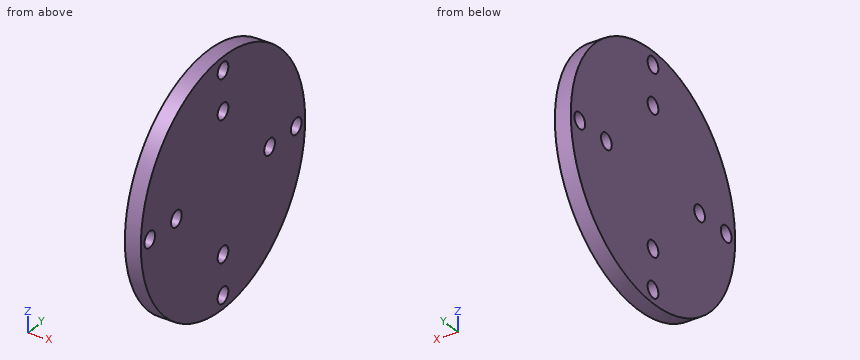
from build123d import *

# Parameters (mm, degrees)
SKETCH1_R           = 23
SKETCH1_R_2         = 1.5
BOSS_EXTRUDE1_DEPTH = 3


with BuildPart() as part:
    # Sketch1 → Boss-Extrude1 (new body)
    with BuildSketch(Plane(origin=(0, 0, 0), x_dir=(0, 0, -1), z_dir=(1, 0, 0))):
        with Locations((0, 16.5)):
            Circle(SKETCH1_R)
        with Locations((0, -4)):
            Circle(SKETCH1_R_2, mode=Mode.SUBTRACT)
        with Locations((0, 3.46)):
            Circle(SKETCH1_R_2, mode=Mode.SUBTRACT)
        with Locations((-13.04, 16.5)):
            Circle(SKETCH1_R_2, mode=Mode.SUBTRACT)
        with Locations((-20.5, 16.5)):
            Circle(SKETCH1_R_2, mode=Mode.SUBTRACT)
        with Locations((0, 29.54)):
            Circle(SKETCH1_R_2, mode=Mode.SUBTRACT)
        with Locations((0, 37)):
            Circle(SKETCH1_R_2, mode=Mode.SUBTRACT)
        with Locations((13.04, 16.5)):
            Circle(SKETCH1_R_2, mode=Mode.SUBTRACT)
        with Locations((20.5, 16.5)):
            Circle(SKETCH1_R_2, mode=Mode.SUBTRACT)
    extrude(amount=BOSS_EXTRUDE1_DEPTH)


solid = part.part
The listing builds one solid part. Answer for the finished solid, in the listing's coordinates (mm). Coordinates: 2 decimals unless noted, no trailing zeros. Order: outer loops, then holes, each group sorted by start corner. A loop starts at its lowest first (then second) coordinate and runs counter-clockwise, first axis right, second up. Notation, with made-up numbers: M -39.5,85.5 L -28.5,85.5 A14 cw -28.5,106.5 Z; hole C -10.5,21 d4. An arc over 180 degrees is marked long. Use CSV: the item, a comma, the result in double quotes.
Q1. Section B-B (x = 0.65) is taken. Give the number of separate pieces and of enclosed holes in the cut face, then the cut area to 3 significant figures.
Here are the results:
separate pieces,"1"
enclosed holes,"8"
area,"1,610 mm2"
Q2. Section C-C (z = -20.5) is taken. Determine the outline of the cut face in (x, y).
Here are the results:
outline,"M 0,6.07 L 3,6.07 L 3,15 L 0,15 Z; M 0,18 L 3,18 L 3,26.93 L 0,26.93 Z"
Q3. Section D-D (y = -4) is taken. Determine the outline of the cut face in (x, z), then the cut area to 3 significant figures.
Here are the results:
outline,"M 0,-10.43 L 3,-10.43 L 3,-1.5 L 0,-1.5 Z; M 0,1.5 L 3,1.5 L 3,10.43 L 0,10.43 Z"
area,"53.6 mm2"
Q4. Section A-A (y = 16.5) is taken. Determine the outline of the cut face in (x, z), then the cut area to 3 significant figures.
Here are the results:
outline,"M 0,-23 L 3,-23 L 3,-22 L 0,-22 Z; M 0,-19 L 3,-19 L 3,-14.54 L 0,-14.54 Z; M 0,-11.54 L 3,-11.54 L 3,11.54 L 0,11.54 Z; M 0,14.54 L 3,14.54 L 3,19 L 0,19 Z; M 0,22 L 3,22 L 3,23 L 0,23 Z"
area,"102 mm2"
Q5. Straight lines are drawn through the part: L1, parallel to Y at x = 2.25, z = 0; L2, parallel to Z at x = 0.8, y = 16; L3, parallel to Y at x = 2.85, z = -0.5. For each, find the intervals that lie inside material, in ascending order.
Here are the results:
L1,"-6.5 to -5.5, -2.5 to 1.96, 4.96 to 28.04, 31.04 to 35.5, 38.5 to 39.5"
L2,"-22.99 to -21.91, -19.09 to -14.45, -11.63 to 11.63, 14.45 to 19.09, 21.91 to 22.99"
L3,"-6.49 to -5.41, -2.59 to 2.05, 4.87 to 28.13, 30.95 to 35.59, 38.41 to 39.49"
